Could you check a few things on this model? Use its own coordinates, in mm. Give positions to 0.01 mm unless a question says otherwise; leave off trailing zeros. One line per item, written item: value. Start each with the question number.
Q1. If I drill on line 1 (Y direction, x = 0, z = 5.75); line 2 (X direction, y = 0.5, z = 4.75); line 3 (Y direction, x = -41.5, z = 1.75), over which ranges is the centre line in solid material (lowest first)? Write a range as from..to.
Q2. I'm going to push flat-ended pins straight in: P1, Ø1, axis at x = 53.5, z = 8.5, coming from the -Y side; P2, Ø6, axis at x = -40, z = 2, coming from the -Y side; P3, Ø2, axis at x = -33.5, y = 157, coming from the -Z side. Where does each tip first touch, or does it pass through?
Q3. If we mould it in two halves opening along Y, with no side actions, what happens to faces 1 (the face through (1, 237, 5)), 2 (the face through (-70, 163, 5)), 3 (the face through (1.08, -4.88, 4.93))? For each: released by +Y, released by -Y, zero draft, split by the parting line, or undercut.
```python
from build123d import *

# Parameters (mm, degrees)
BOSS_EXTRUDE1_DEPTH = 10
SKETCH2_R           = 5
CUT_EXTRUDE1_DEPTH  = 10


with BuildPart() as part:
    # Sketch1 → Boss-Extrude1 (new body)
    with BuildSketch(Plane.XY):
        with BuildLine():
            Line((70, 87), (70, 237))
            Line((70, 237), (-70, 237))
            Line((-70, 237), (-70, 87))
            add(Edge.make_bspline(
                [(0, -13), (-4.605948028, -10.653982198), (-21.385528158, -2.10738257), (-9.908182864, 31.191471557), (-24.240732749, 61.889747712), (-47.857626179, 72.570821606), (-70, 76.647728673), (-70, 87)],
                knots=[0, 0, 0, 0, 0.050956587, 0.18563608, 0.29003014, 0.381689368, 0.470019459, 0.470019459, 0.470019459, 0.470019459], degree=3))
            add(Edge.make_bspline(
                [(0, -13), (4.605948028, -10.653982198), (21.385528158, -2.10738257), (9.908182864, 31.191471557), (24.240732749, 61.889747712), (47.857626179, 72.570821606), (70, 76.647728673), (70, 87)],
                knots=[0, 0, 0, 0, 0.050956587, 0.18563608, 0.29003014, 0.381689368, 0.470019459, 0.470019459, 0.470019459, 0.470019459], degree=3))
        make_face()
    extrude(amount=BOSS_EXTRUDE1_DEPTH)

    # Sketch2 → Cut-Extrude1 (cut)
    with BuildSketch(Plane(origin=(0, 0, 0), x_dir=(-1, 0, 0), z_dir=(0, 0, -1))):
        Circle(SKETCH2_R)
    extrude(amount=-CUT_EXTRUDE1_DEPTH, mode=Mode.SUBTRACT)


solid = part.part
```
Worked answers:
1. line 1: y = -13..-5, 5..237
1. line 2: x = -14.91..-4.97, 4.97..14.91
1. line 3: y = 69.11..237
2. P1: stops at y = 72.85
2. P2: stops at y = 67.07
2. P3: stops at z = 0
3. face 1: released by +Y
3. face 2: zero draft
3. face 3: undercut
